```python
from build123d import *

# Parameters (mm, degrees)
SKETCH1_W           = 120
SKETCH1_H           = 55
BOSS_EXTRUDE1_DEPTH = 5
SKETCH2_W           = 120
SKETCH2_H           = 7.5
BOSS_EXTRUDE2_DEPTH = 20
SKETCH3_W           = 120
SKETCH3_H           = 2.5
BOSS_EXTRUDE4_DEPTH = 20
BOSS_EXTRUDE5_DEPTH = 190
SKETCH9_W           = 310
SKETCH9_H           = 25
BOSS_EXTRUDE6_DEPTH = 70
SKETCH14_R          = 5.5
CUT_EXTRUDE5_DEPTH  = 153
SKETCH15_W          = 125
SKETCH15_H          = 25
CUT_EXTRUDE6_DEPTH  = 190


with BuildPart() as part:
    # Sketch1 → Boss-Extrude1 (new body)
    with BuildSketch(Plane(origin=(0, 0, 0), x_dir=(1, 0, 0), z_dir=(0, 1, 0))):
        Rectangle(SKETCH1_W, SKETCH1_H)
    extrude(amount=BOSS_EXTRUDE1_DEPTH)

    # Sketch2 → Boss-Extrude2 (add)
    with BuildSketch(Plane(origin=(0, 5, 0), x_dir=(1, 0, 0), z_dir=(0, 1, 0))):
        with Locations((0, -23.75)):
            Rectangle(SKETCH2_W, SKETCH2_H)
    extrude(amount=BOSS_EXTRUDE2_DEPTH)

    # Sketch3 → Boss-Extrude4 (add)
    with BuildSketch(Plane(origin=(0, 5, 0), x_dir=(1, 0, 0), z_dir=(0, 1, 0))):
        with Locations((0, 26.25)):
            Rectangle(SKETCH3_W, SKETCH3_H)
    extrude(amount=BOSS_EXTRUDE4_DEPTH)

    # Sketch8 → Boss-Extrude5 (add)
    with BuildSketch(Plane.ZY.offset(60)):
        Polygon((-27.5, 0), (-27.5, 25), (-25, 25), (-25, 5), (20, 5), (20, 25), (27.5, 25), (27.5, 0), align=None)
    extrude(amount=BOSS_EXTRUDE5_DEPTH)

    # Sketch9 → Boss-Extrude6 (add)
    with BuildSketch(Plane(origin=(0, 0, -27.5), x_dir=(-1, 0, 0), z_dir=(0, 0, -1))):
        with Locations((95, 12.5)):
            Rectangle(SKETCH9_W, SKETCH9_H)
    extrude(amount=BOSS_EXTRUDE6_DEPTH)

    # Sketch14 → Cut-Extrude5 (cut)
    with BuildSketch(Plane(origin=(0, 0, 0), x_dir=(-1, 0, 0), z_dir=(0, -1, 0))):
        with Locations(Location((225.445279058, 7.255161462, 0), (0, 0, 90))):
            Circle(SKETCH14_R)
        with Locations(Location((175.445279058, 7.255161462, 0), (0, 0, 90))):
            Circle(SKETCH14_R)
        with Locations(Location((225.445279058, 57.255161462, 0), (0, 0, 90))):
            Circle(SKETCH14_R)
        with Locations(Location((148.0182107, 48.5, 0), (0, 0, 90))):
            Circle(SKETCH14_R)
        with Locations(Location((183.240850763, 83.987541856, 0), (0, 0, 90))):
            Circle(SKETCH14_R)
    extrude(amount=-CUT_EXTRUDE5_DEPTH, mode=Mode.SUBTRACT)

    # Sketch15 → Cut-Extrude6 (cut)
    with BuildSketch(Plane(origin=(60, 0, 0), x_dir=(0, 0, -1), z_dir=(1, 0, 0))):
        with Locations((35, 12.5)):
            Rectangle(SKETCH15_W, SKETCH15_H)
    extrude(amount=-CUT_EXTRUDE6_DEPTH, mode=Mode.SUBTRACT)


solid = part.part
```
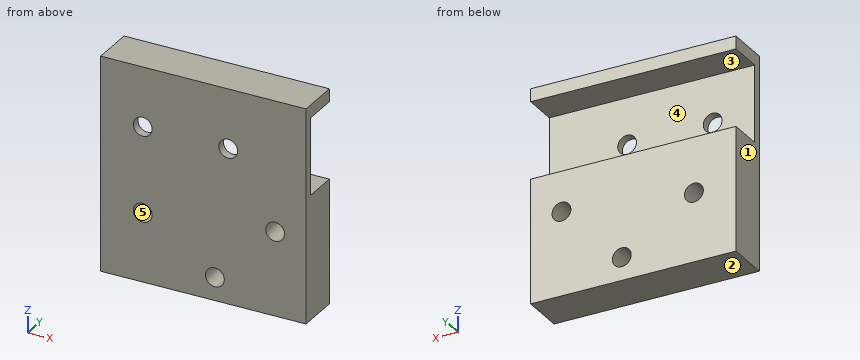
Verification items for the finished model (mm, model axes). Face numbers are marked on the shaded views. A direction names the side the tool comes from. Give positions to 0.01 mm unless a question says otherwise; leave off trailing zeros. Loops run counter-clockwise (first coordinate to the right, second up) from the corner with the lowest first, then second, coordinate; pieces in that order, holes last. Notation, with made-up numbers: M -33.75,5.5 L 20.25,5.5 A23 cw 20.25,22.5 Z; hole C -38.5,-31 d2. An arc over 180 degrees is marked long. Return JSON: item names as keys, results as strings.
1) Section check C-C, the plane y = 11.75. Enter the section's corners in (x, z).
Findings:
{"outline": "M -250,-97.5 L -130,-97.5 L -130,-25 L -250,-25 Z; M -250,20 L -130,20 L -130,27.5 L -250,27.5 Z; hole C -225.45,-57.26 d11; hole C -183.24,-83.99 d11; hole C -148.02,-48.5 d11"}
2) Section check A-A, the plane z = -48.5. Enter the section's corners in (x, y).
Findings:
{"outline": "M -250,0 L -153.52,0 L -153.52,25 L -250,25 Z; M -142.52,0 L -130,0 L -130,25 L -142.52,25 Z"}
3) Material ranges on L1, parallel to Z at x = -225, y = 6.25; L2, parallel to Z at x = -140.5, y = 9.75; L3, parallel to Z at x = -187.5, y = 15, recorded low to high. Write a range as [from, to].
Findings:
{"L1": "z = [-97.5, -62.74], [-51.77, -25], [20, 27.5]", "L2": "z = [-97.5, -25], [20, 27.5]", "L3": "z = [-97.5, -87.47], [-80.51, -25], [20, 27.5]"}
4) Section check D-D, the plane z = 16. Enter the section's corners in (x, y).
Findings:
{"outline": "M -250,0 L -130,0 L -130,5 L -250,5 Z"}
5) Mould release check, pull along Z, two halves, no side actions. Record for the marked faces 1, 2 and 3: released by +Z, released by -Z, zero draft, split by the parting line, or undercut.
Findings:
{"face 1": "zero draft", "face 2": "released by -Z", "face 3": "undercut"}
6) Gauge pin test, flat end, axial feed: P1, Ø14.5, axis at x = -225.45, z = -7.26, coming from the +Y side. Record the tip position at first contact, or that the pin passes through.
Findings:
{"P1": "stops at y = 5"}
7) Tool access check on the marked faces 4 and 5. Record the directions out of +Z, -Z, +X, -X, +Y, -Y that give a thin tool (end or side, any length) a straight path to the whole face; none if there is none.
Findings:
{"face 4": "+X, -X, +Y", "face 5": "+Y, -Y"}
8) Section check B-B, the plane x = -165. Enter the section's corners in (y, z).
Findings:
{"outline": "M 0,-97.5 L 25,-97.5 L 25,-25 L 5,-25 L 5,20 L 25,20 L 25,27.5 L 0,27.5 Z"}
